Build history of the part. All positions in model axes, mm. Give positions to 0.01 mm unless a question says otherwise; leave off trailing zeros. Order: outer loops, then holes, each group sorted by start corner. A loop starts at its lowest first (then second) coordinate and runs counter-clockwise, first axis right, second up. Notation, with made-up numbers: M 83.5,83 L 106.5,83 A23 ccw 106.5,95 Z; hole C 76.25,65 d11. An arc over 180 degrees is marked long. Use CSV: the item, a comma, the result in double quotes. Start each with the question number.
Item 1: Wall check: line 1 along Y through (x, z) = (6, 1); line 2 along X through (y, z) = (-16.5, -29.5); line 3 along Y through (x, z) = (3.75, 1.5). Give the ranges that are in metal, low to high.
Item 2: Pin check, flat tips, straight feed: P1, Ø0.9, axis at y = 9, z = 17, coming from the +X side; P2, Ø0.9, axis at y = -16, z = -12, coming from the +X side; P3, Ø13, axis at x = -11.5, z = -25.5, coming from the +Y side. Stop position of each tip, or through.
Item 3: Band-saw the part on A-A on y = -1. Write the cut outline in (x, z), plus the area to 3 significant figures.
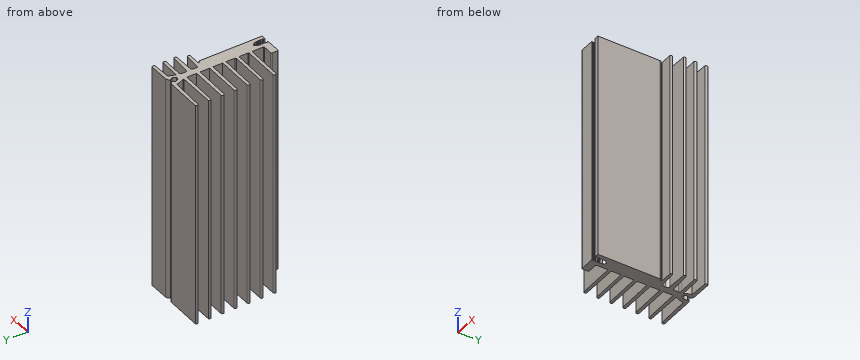
from build123d import *

# Parameters (mm, degrees)
F1_DEPTH      = 50.8
F1_DEPTH_BACK = 50.8


# Not quite as in the source:
# - a feature of the source that left no trace in its solid (it failed there, or was rolled back) is left out
# - the program builds the solid bodies; features that only make, move or delete a surface that nothing else refers to are left out


with BuildPart() as f1:
    # F0 (on Top) → F1 (new body, two sides)
    with BuildSketch(Plane.XY) as f1_sk:
        with BuildLine():
            Line((-3.3736736514, 24.7951317579), (-19.627969712, 24.8093213886))
            ThreePointArc((-19.627969712, 24.8093213886), (-20.0021253233, 24.2030567982), (-19.6617264301, 23.57721515))
            Line((-19.6617264301, 23.57721515), (-4.5088279332, 23.1754036615))
            ThreePointArc((-4.5088279332, 23.1754036615), (-4.1624050394, 21.325828975), (-3.3758739325, 19.6163541549))
            Line((-3.3758739325, 19.6163541549), (-3.3873883076, 19.2034132779))
            Line((-3.3873883076, 19.2034132779), (-19.6617264301, 18.969476223))
            ThreePointArc((-19.6617264301, 18.969476223), (-20.0032717352, 18.3534221724), (-19.6617264301, 17.7373681217))
            Line((-19.6617264301, 17.7373681217), (-2.9635052222, 17.5993758319))
            Line((-2.9635052222, 17.5993758319), (-3.0178399757, 13.2140200585))
            Line((-3.0178399757, 13.2140200585), (-19.4929447025, 13.2140200585))
            ThreePointArc((-19.4929447025, 13.2140200585), (-20.0233587748, 12.5220152549), (-19.4929447025, 11.8300104514))
            Line((-19.4929447025, 11.8300104514), (-3.0178399757, 11.6258831695))
            Line((-3.0178399757, 11.6258831695), (-3.0178399757, 7.360490039))
            Line((-3.0178399757, 7.360490039), (-19.4929447025, 7.360490039))
            ThreePointArc((-19.4929447025, 7.360490039), (-20.0219986391, 6.7022417206), (-19.4929447025, 6.0439934023))
            Line((-19.4929447025, 6.0439934023), (-2.9621112743, 5.8546986264))
            Line((-2.9621112743, 5.8546986264), (-3.0178399757, 1.493252581))
            Line((-3.0178399757, 1.493252581), (-19.4929447025, 1.493252581))
            ThreePointArc((-19.4929447025, 1.493252581), (-19.999079636, 0.8518822287), (-19.4929447025, 0.2105118765))
            Line((-19.4929447025, 0.2105118765), (-3.0178399757, 0))
            Line((-3.0178399757, 0), (-3.0178399757, -3.950452432))
            Line((-3.0178399757, -3.950452432), (-3.3726599067, -4.3803495355))
            Line((-3.3726599067, -4.3803495355), (-19.4929447025, -4.3803495355))
            ThreePointArc((-19.4929447025, -4.3803495355), (-20.0026487971, -5.0217199605), (-19.4929447025, -5.6630903855))
            Line((-19.4929447025, -5.6630903855), (-3.3726599067, -5.7729091495))
            Line((-3.3726599067, -5.7729091495), (-3.0178399757, -6.1277290806))
            Line((-3.0178399757, -6.1277290806), (-3.0178399757, -9.7752762958))
            Line((-3.0178399757, -9.7752762958), (-3.2525765998, -10.18643938))
            Line((-3.2525765998, -10.18643938), (-19.4929447025, -10.18643938))
            ThreePointArc((-19.4929447025, -10.18643938), (-20.0181876942, -10.8531266451), (-19.4929447025, -11.5198139101))
            Line((-19.4929447025, -11.5198139101), (-3.2525765998, -11.6145808049))
            Line((-3.2525765998, -11.6145808049), (-3.0190503156, -11.9383819401))
            Line((-3.0190503156, -11.9383819401), (-3.0190503156, -16.7704734888))
            Line((-3.0190503156, -16.7704734888), (-3.3736736514, -17.0262288302))
            Line((-3.3736736514, -17.0262288302), (-7.4309431948, -17.0262288302))
            ThreePointArc((-7.4309431948, -17.0262288302), (-7.7883055211, -17.1251856492), (-7.9560680315, -17.4558758736))
            Line((-7.9560680315, -17.4558758736), (-7.9560680315, -19.7419915348))
            ThreePointArc((-7.9560680315, -19.7419915348), (-7.8385182356, -20.0781647595), (-7.497502665, -20.1808232814))
            Line((-7.497502665, -20.1808232814), (-1.1584198955, -20.1714233881))
            Line((-1.1584198955, -20.1714233881), (-1.138712159, -19.8357657809))
            Line((-1.138712159, -19.8357657809), (-1.4197152341, -19.5692516863))
            Line((-1.4197152341, -19.5692516863), (-1.160888255, -19.2963536351))
            Line((-1.160888255, -19.2963536351), (-1.138712159, -18.9265421938))
            Line((-1.138712159, -18.9265421938), (-1.3017905422, -18.7004221842))
            Line((-1.3017905422, -18.7004221842), (-1.0179714863, -18.4957310875))
            Line((-1.0179714863, -18.4957310875), (-1.018282466, -17.9434493202))
            Line((-1.018282466, -17.9434493202), (-1.4397868638, -17.7126266085))
            Line((-1.4397868638, -17.7126266085), (-1.138712159, -17.3513367812))
            Line((-1.138712159, -17.3513367812), (-1.138712159, -16.8896894959))
            Line((-1.138712159, -16.8896894959), (-1.4169517005, -16.588565616))
            Line((-1.4169517005, -16.588565616), (-1.138712159, -16.3878984806))
            Line((-1.138712159, -16.3878984806), (-1.138712159, -15.3241008577))
            Line((-1.138712159, -15.3241008577), (0, -14.1900535673))
            Line((0, -14.1900535673), (1.0927112374, -15.4159043089))
            Line((1.0927112374, -15.4159043089), (1.1339221451, -16.1570739001))
            Line((1.1339221451, -16.1570739001), (1.3667184391, -16.3108690956))
            Line((1.3667184391, -16.3108690956), (1.0229069001, -16.558826939))
            Line((1.0229069001, -16.558826939), (1.0490959976, -17.0602984726))
            Line((1.0490959976, -17.0602984726), (1.462081531, -17.337922364))
            Line((1.462081531, -17.337922364), (1.1371706318, -17.572249013))
            Line((1.1371706318, -17.572249013), (1.1339221451, -18.033772707))
            Line((1.1339221451, -18.033772707), (1.4404929399, -18.274631373))
            Line((1.4404929399, -18.274631373), (1.1339221451, -18.4957310875))
            Line((1.1339221451, -18.4957310875), (1.1293826392, -19.1477481276))
            Line((1.1293826392, -19.1477481276), (1.5007078182, -19.3585008383))
            Line((1.5007078182, -19.3585008383), (1.1495453005, -19.6058004949))
            Line((1.1495453005, -19.6058004949), (1.1458612277, -20.178947635))
            Line((1.1458612277, -20.178947635), (2.9662006887, -20.178947635))
            Line((2.9662006887, -20.178947635), (2.9662006887, 7.7263202994))
            Line((2.9662006887, 7.7263202994), (2.825798234, 8.2537010312))
            Line((2.825798234, 8.2537010312), (2.1506715566, 8.2537010312))
            Line((2.1506715566, 8.2537010312), (2.1506715566, 9.0581281111))
            Line((2.1506715566, 9.0581281111), (7.5833620504, 9.0581281111))
            ThreePointArc((7.5833620504, 9.0581281111), (8.0257459726, 9.6480058962), (7.5632906519, 10.222283192))
            Line((7.5632906519, 10.222283192), (0.0440248574, 10.6278444304))
            Line((0.0440248574, 10.6278444304), (0, 11.1270683113))
            Line((0, 11.1270683113), (-0.1044616438, 12.3116206378))
            ThreePointArc((-0.1044616438, 12.3116206378), (0.126172228, 13.1274286151), (0.8690126706, 13.5359903798))
            Line((0.8690126706, 13.5359903798), (9.5102395862, 13.8351768255))
            ThreePointArc((9.5102395862, 13.8351768255), (9.9020840969, 14.4295718757), (9.570454247, 15.0595474616))
            Line((9.570454247, 15.0595474616), (0.6003075975, 15.5130466074))
            ThreePointArc((0.6003075975, 15.5130466074), (0.2149232739, 15.60577238), (0, 15.9388296306))
            Line((0, 15.9388296306), (0, 18.1245207787))
            ThreePointArc((0, 18.1245207787), (0.2171557282, 18.5044688755), (0.6286933785, 18.6533108354))
            Line((0.6286933785, 18.6533108354), (9.570454247, 18.6533108354))
            ThreePointArc((9.570454247, 18.6533108354), (9.9234885577, 19.2956030182), (9.570454247, 19.9378952011))
            Line((9.570454247, 19.9378952011), (0.3673353055, 20.0769044086))
            Line((0.3673353055, 20.0769044086), (0.3164518273, 20.2818233147))
            ThreePointArc((0.3164518273, 20.2818233147), (0.9977498793, 21.6728398839), (1.3667184391, 23.1771524623))
            Line((1.3667184391, 23.1771524623), (9.570454247, 23.5285814479))
            ThreePointArc((9.570454247, 23.5285814479), (9.9232117791, 24.1969227418), (9.570454247, 24.8652640357))
            Line((9.570454247, 24.8652640357), (0.5151510704, 24.7951317579))
            ThreePointArc((0.5151510704, 24.7951317579), (-0.4052105617, 24.3861366082), (-0.9608993423, 23.5461648554))
            Line((-0.9608993423, 23.5461648554), (-0.1758071594, 22.2885161638))
            Line((-0.1758071594, 22.2885161638), (-0.8712234916, 20.8444888061))
            Line((-0.8712234916, 20.8444888061), (-2.148604719, 20.8550449461))
            Line((-2.148604719, 20.8550449461), (-2.9008225538, 22.3878659308))
            Line((-2.9008225538, 22.3878659308), (-2.3517927621, 23.5461648554))
            ThreePointArc((-2.3517927621, 23.5461648554), (-2.6533703145, 24.3419450304), (-3.3736736514, 24.7951317579))
        make_face()
    extrude(amount=F1_DEPTH)
    extrude(f1_sk.sketch, amount=-F1_DEPTH_BACK)


solid = f1.part
Model answer:
1,line 1,"y = 9.06 to 10.31, 13.71 to 15.24, 18.65 to 19.99, 23.38 to 24.84"
1,line 2,"x = -3.02 to -1.29, 1.1 to 2.97"
1,line 3,"y = 9.06 to 10.43, 13.64 to 15.35, 18.65 to 20.03, 23.28 to 24.82"
2,P1,"stops at x = 8"
2,P2,"stops at x = 2.97"
2,P3,"stops at y = 24.81"
3,outline,"M -3.02,-50.8 L 2.97,-50.8 L 2.97,50.8 L -3.02,50.8 Z"
3,area,"608 mm^2"
